Solid Edge part; units mm, degrees
sketch "Sketch1" plane through (0, 0, 0) normal (0, 0, 1) x (1, 0, 0)
  line L0 (0, -86.6025) -> (75, 43.3013)
  line L1 (75, 43.3013) -> (-75, 43.3013)
  line L2 (-75, 43.3013) -> (0, -86.6025)
extrude "Protrusion1" add sketch "Sketch1" along normal up to vertex (122.4745 mm away)
sketch "Sketch2" plane through (0, 0, 0) normal (1, 0, 0) x (0, 1, 0)
  line L0 (0, 122.4745) -> (43.3013, 0)
extrude "Cutout1" cut sketch "Sketch2" along normal mid plane 491.8403 material side at (0, 21.6978, 61.2539)
pattern_circular "Pattern1" count 3 over 360 about axis through (0, 0, 122.4745) along (0, 0, -1) of "Cutout1"
Here's how the part is built. I have some questions about the finished solid (model axes, mm). Give positions to 0.01 mm unless a question says otherwise; leave off trailing zeros. Loops run counter-clockwise (first coordinate to the right, second up) from the corner with the lowest first, then second, coordinate; pieces in that order, holes last. Notation, with made-up numbers: M 32,19 L 71,19 A28 ccw 71,57 Z; hole C 16,87 d7. An arc over 180 degrees is marked long. Use one line per item in the form item = value. Start each with the question number.
Q1. Will these pins go through, and if not, where does the flat tip stop? pin 1 Ø12 at (y, z) = (-23.5, 103) entering from -X; pin 2 Ø1 at (x, z) = (-26, 51) entering from -Y; pin 3 Ø1.5 at (x, z) = (38.5, 55) entering from -Y; pin 4 Ø10 at (x, z) = (36, 59.5) entering from +Y.
Q2. If we section it at B-B (z = 48): Write out the boundary of the cut face in (x, y).
Q3. I need wall thicknesses on line 1 along Z through (x, y) = (-30, -7); line 2 along Y through (x, z) = (-7, 72); line 3 along Y through (x, z) = (-10.5, 20.5). Which ranges of each line are inside material? Lowest first, please.
Taken from the geometry:
q1.pin_1 = through
q1.pin_2 = -6.44
q1.pin_3 = 17.57
q1.pin_4 = 24.03
q2.outline = M -45.61,26.33 L 0,-52.66 L 45.61,26.33 Z
q3.line_1 = 0 to 39.09
q3.line_2 = -23.57 to 17.85
q3.line_3 = -53.92 to 36.05
